```python
from build123d import *

# Parameters (mm, degrees)
SKETCH1_R                    = 1.5875
MAINPCB_DEPTH                = 2.54
SKETCH2_W                    = 12.7
SKETCH2_H                    = 47.625
CHARGER_USBCONNECTIONS_DEPTH = 9.525
SKETCH3_W                    = 66.675
SKETCH3_H                    = 4.7625
GPIO_HEADER_DEPTH            = 9.525


with BuildPart() as part:
    # Sketch1 → MainPCB (new body)
    with BuildSketch(Plane(origin=(0, 0, 0), x_dir=(1, 0, 0), z_dir=(0, 1, 0))):
        with BuildLine():
            Line((-46.0375, 31.75), (46.0375, 31.75))
            ThreePointArc((46.0375, 31.75), (48.28256403, 30.82006403), (49.2125, 28.575))
            Line((49.2125, 28.575), (49.2125, -28.575))
            ThreePointArc((49.2125, -28.575), (48.28256403, -30.82006403), (46.0375, -31.75))
            Line((46.0375, -31.75), (-46.0375, -31.75))
            ThreePointArc((-46.0375, -31.75), (-48.28256403, -30.82006403), (-49.2125, -28.575))
            Line((-49.2125, -28.575), (-49.2125, 28.575))
            ThreePointArc((-49.2125, 28.575), (-48.28256403, 30.82006403), (-46.0375, 31.75))
        make_face()
        with Locations((-46.0375, 28.575)):
            Circle(SKETCH1_R, mode=Mode.SUBTRACT)
        with Locations((46.0375, 28.575)):
            Circle(SKETCH1_R, mode=Mode.SUBTRACT)
        with Locations((46.0375, -28.575)):
            Circle(SKETCH1_R, mode=Mode.SUBTRACT)
        with Locations((-46.0375, -28.575)):
            Circle(SKETCH1_R, mode=Mode.SUBTRACT)
    extrude(amount=MAINPCB_DEPTH)

    # Sketch2 → Charger_USBConnections (add)
    with BuildSketch(Plane(origin=(0, 2.54, 0), x_dir=(1, 0, 0), z_dir=(0, 1, 0))):
        with Locations((-42.8625, 1.5875)):
            Rectangle(SKETCH2_W, SKETCH2_H)
    extrude(amount=CHARGER_USBCONNECTIONS_DEPTH)

    # Sketch3 → GPIO Header (add)
    with BuildSketch(Plane(origin=(0, 2.54, 0), x_dir=(1, 0, 0), z_dir=(0, 1, 0))):
        with Locations((0, 24.60625)):
            Rectangle(SKETCH3_W, SKETCH3_H)
    extrude(amount=GPIO_HEADER_DEPTH)


solid = part.part
```
Geometry check sheet. Reference: the model listing, model coordinates, mm. A direction names the side the tool comes from. Coordinates: 2 decimals unless noted, no trailing zeros. Order: outer loops, then holes, each group sorted by start corner. A loop starts at its lowest first (then second) coordinate and runs counter-clockwise, first axis right, second up. Notation, with made-up numbers: M 47,-3.75 L 96,-3.75 A21 ccw 96,9.25 Z; hole C 88,15.5 d6. An arc over 180 degrees is marked long. One line per question, with ' | ' between items. Start each with the question number.
Item 1: Cross-section at C-C on z = 11.5. Enter the section's corners in (x, y) (1 decimal), then the cut area to 3 significant figures.
Item 2: Gauge pin test, flat ends, axial feed: pin 1 (2 mm diameter, centred on x = -36.5, y = 8.5, fed in from +Z) (3 decimals); pin 2 (3.5 mm diameter, centred on x = 46.04, z = 28.58, fed in from +Y); pin 3 (5 mm diameter, centred on x = -31.5, z = -12.5, fed in from -Y); pin 4 (2.5 mm diameter, centred on y = 8, z = -26, fed in from +X). Record the tip position at first contact, or that the pin passes through.
Item 3: Cross-section at D-D on x = 43. Enter the section's corners in (y, z).
Item 4: Material ranges on L1, parallel to Y at x = 35.5, z = 19; L2, parallel to X at y = 3.75, z = 10.5; L3, parallel to Z at x = 0, y = 11.5 (1 decimal), recorded low to high. Write a range as [from, to].
Item 5: Cross-section at A-A on y = 7.25. Enter the section's corners in (x, z) (1 decimal), then the cut area to 3 significant figures.
Item 6: Set-up check for faces 5 (the flat face through (0, 7, -22.225)), 6 (the flat face through (0, 7, -26.988)), 7 (the flat face through (-43, 7, -25.4)), 8 (the cylindrical face through (48.3, 1.3, -30.8)), 9 (the flat face through (33.338, 7, -25)): record each of +Z, -Z, +X, -X, +Y, -Y from which the full face is reachable in a straight line by a thin tool's end or side.
Item 7: Draft check along X on faces 1 (the cylindrical face through (-45.18, 1.25, 27.24)), 2 (the cylindrical face through (-48.3, 1.3, -30.8)), 3 (the flat face through (-43, 7, 22.225)), 4 (the cylindrical face through (46.891, 1.252, 27.236)). Enter one of: pulls with the +X half, pulls with the -X half, needs draft (parallel to the pull), parting line crosses it, or undercut.
Findings:
1) outline: M -49.2,0 L 49.2,0 L 49.2,2.5 L -36.5,2.5 L -36.5,12.1 L -49.2,12.1 Z | area: 371 mm²
2) pin 1: stops at z = 22.225 | pin 2: stops at y = 2.54 | pin 3: stops at y = 0 | pin 4: stops at x = 33.34
3) outline: M 0,-31.75 L 2.54,-31.75 L 2.54,31.75 L 0,31.75 Z
4) L1: y = [0, 2.54] | L2: x = [-49.21, -36.51] | L3: z = [-27, -22.2]
5) outline: M -49.2,-25.4 L -36.5,-25.4 L -36.5,22.2 L -49.2,22.2 Z; M -33.3,-27 L 33.3,-27 L 33.3,-22.2 L -33.3,-22.2 Z | area: 922 mm²
6) face 5: +Z, +X, +Y | face 6: -Z, +X, -X, +Y | face 7: -Z, -X, +Y | face 8: -Z, +X, +Y, -Y | face 9: +Z, -Z, +X, +Y
7) face 1: undercut | face 2: pulls with the -X half | face 3: needs draft | face 4: undercut
